from build123d import *

# Parameters (mm, degrees)
F0_W      = 50
F0_H      = 80
F1_DEPTH  = 3
F2_W      = 50
F2_H      = 4
F3_DEPTH  = 40
F2_H_2    = 9
F4_DEPTH  = 30
F5_W      = 25
F5_H      = 5
F6_DEPTH  = 12.5
F8_DEPTH  = 9
F9_R      = 1.5
F10_DEPTH = 3
F7_R      = 2.85
F11_DEPTH = 78
F7_R_2    = 5
F12_DEPTH = 80
F13_R     = 1.5
F14_DEPTH = 4


with BuildPart() as f1:
    # F0 (on Front) → F1 (new body)
    with BuildSketch(Plane.XZ):
        with Locations((25, 40)):
            Rectangle(F0_W, F0_H)
    extrude(amount=F1_DEPTH)

    # F2 (on face) → F3 (join)
    with BuildSketch(Plane.XZ.offset(3)):
        with Locations((25, 2)):
            Rectangle(F2_W, F2_H)
    extrude(amount=F3_DEPTH)

    # F2 (on face) → F4 (join)
    with BuildSketch(Plane.XZ.offset(3)):
        with Locations((25, 75.5)):
            Rectangle(F2_W, F2_H_2)
    extrude(amount=F4_DEPTH)

    # F5 (on face) → F6 (cut)
    with BuildSketch(Plane.XZ.offset(33)):
        with Locations((25, 75.5)):
            Rectangle(F5_W, F5_H)
    extrude(amount=-F6_DEPTH, mode=Mode.SUBTRACT)

    # F7 (on face) → F8 (cut)
    with BuildSketch(Plane.XY.offset(80)):
        with BuildLine():
            Line((16, -33), (34, -33))
            ThreePointArc((34, -33), (25, -24), (16, -33))
        make_face()
    extrude(amount=-F8_DEPTH, mode=Mode.SUBTRACT)

    # F9 (on face) → F10 (cut)
    with BuildSketch(Plane.XZ.offset(33)):
        with Locations((5, 75.5)):
            Circle(F9_R)
        with Locations((45, 75.5)):
            Circle(F9_R)
    extrude(amount=-F10_DEPTH, mode=Mode.SUBTRACT)

    # F7 (on face) → F11 (cut)
    with BuildSketch(Plane.XY.offset(80)):
        with Locations((9, -14)):
            Circle(F7_R)
        with Locations((41, -14)):
            Circle(F7_R)
    extrude(amount=-F11_DEPTH, mode=Mode.SUBTRACT)

    # F7 (on face) → F12 (cut)
    with BuildSketch(Plane.XY.offset(80)):
        with Locations((25, -14)):
            Circle(F7_R_2)
    extrude(amount=-F12_DEPTH, mode=Mode.SUBTRACT)

    # F13 (on face) → F14 (cut)
    with BuildSketch(Plane.XY.offset(4)):
        with Locations((7, -22)):
            Circle(F13_R)
        with Locations((43, -22)):
            Circle(F13_R)
    extrude(amount=-F14_DEPTH, mode=Mode.SUBTRACT)


solid = f1.part
Verification items for the finished model (mm, model axes). A direction names the side the tool comes from. Round coordinates to 2 decimals unless told otherwise and drop trailing zeros. Loops run counter-clockwise (first coordinate to the right, second up) from the corner with the lowest first, then second, coordinate; pieces in that order, holes last. Notation, with made-up numbers: (69, -1.5) - (112, -1.5) arc R30 cw to (112, 22.5) - close; hole circle Ø7 at (10.25, 48). An arc over 180 degrees is marked (long way). Use a Markdown table: item, result. Add a question column.
1. Section check A-A, the plane y = -22. Record the boundary of the cut face in (x, z).
2. Section check D-D, the plane z = 75.5. Record the boundary of the cut face in (x, y).
3. Access from +Z, -Z, +X, -X, +Y, -Y to the whole of each face (thin tool, end or side, straight path). Record for faces 1 (the face through (25, -20.5, 76)), 2 (the face through (25, -24, 79)), 3 (the face through (25, -23, 4)), 4 (the face through (8, -33, 76)), 5 (the face through (41, -14, 2)).
4. Thickness scan on probe 1 along Z at (x, y) = (45, -32); probe 2 along Z at (x, y) = (47, -12.5); probe 3 along Y at (x, z) = (25, 75). Record the ranges inside material, lowest first. Write a range as [from, to].
5. Section check C-C, the plane y = -14. Give the number of separate pieces and of enclosed holes in the cut face, plus the area to 3 significant figures.
6. Release check for a two-part mould opening along X. For faces 6 (the face through (0, -2, 49)), 7 (the face through (43.718, -13.144, 75.563)), 8 (the face through (25, -21, 71)) record: released by +X, released by -X, zero draft, split by the parting line, or undercut.
7. Gauge pin test, flat ends, axial feed: pin 1 (1.8 mm diameter, centred on x = 43, y = -22, fed in from -Z); pin 2 (4.5 mm diameter, centred on x = 40.5, y = -13.5, fed in from +Z); pin 3 (4.5 mm diameter, centred on x = 38.5, z = 76.5, fed in from -Y); pin 4 (4 mm diameter, centred on x = 26.5, y = -28.5, fed in from +Z). Record the tip position at first contact, or that the pin passes through.
8. Section check B-B, the plane x = 25. Record the boundary of the cut face in (y, z).
Checks:
| question | item | result |
|---|---|---|
| 1 | outline | (0, 0) - (5.5, 0) - (5.5, 4) - (0, 4) - close; (0, 71) - (50, 71) - (50, 80) - (0, 80) - close; (8.5, 0) - (41.5, 0) - (41.5, 4) - (8.5, 4) - close; (44.5, 0) - (50, 0) - (50, 4) - (44.5, 4) - close; hole (12.5, 73) - (37.5, 73) - (37.5, 78) - (12.5, 78) - close |
| 2 | outline | (0, -33) - (3.5, -33) - (3.5, -30) - (6.5, -30) - (6.5, -33) - (12.5, -33) - (12.5, -20.5) - (37.5, -20.5) - (37.5, -33) - (43.5, -33) - (43.5, -30) - (46.5, -30) - (46.5, -33) - (50, -33) - (50, 0) - (0, 0) - close; hole circle Ø5.7 at (9, -14); hole circle Ø10 at (25, -14); hole circle Ø5.7 at (41, -14) |
| 3 | face 1 | -Y |
| 3 | face 2 | +Z, -Y |
| 3 | face 3 | +X, -X, -Y |
| 3 | face 4 | +Z, +X, -X, -Y |
| 3 | face 5 | +Z |
| 4 | probe 1 | z = [0, 4], [71, 74], [77, 80] |
| 4 | probe 2 | z = [0, 4], [71, 80] |
| 4 | probe 3 | y = [-20.5, -19], [-9, 0] |
| 5 | separate pieces | 6 |
| 5 | enclosed holes | 0 |
| 5 | area | 395 mm^2 |
| 6 | face 6 | released by -X |
| 6 | face 7 | undercut |
| 6 | face 8 | zero draft |
| 7 | pin 1 | stops at z = 71 |
| 7 | pin 2 | stops at z = 80 |
| 7 | pin 3 | stops at y = -33 |
| 7 | pin 4 | stops at z = 4 |
| 8 | outline | (-43, 0) - (-19, 0) - (-19, 4) - (-43, 4) - close; (-24, 71) - (-19, 71) - (-19, 80) - (-24, 80) - (-24, 78) - (-20.5, 78) - (-20.5, 73) - (-24, 73) - close; (-9, 0) - (0, 0) - (0, 80) - (-9, 80) - (-9, 71) - (-3, 71) - (-3, 4) - (-9, 4) - close |
